Geometry: see drawing. Coordinates: mm, zero at the bounding-box minimum. A direction names the side the tool comes from. Coordinates: 2 decimals unless noted, no trailing zeros. Loops run counter-clockwise (first coordinate to the right, second up) from the corner with the lowest first, then second, coordinate; pieces in that order, holes last. Notation, with made-up numbers: (73, 11.25) -> (86, 11.25) arc R15 cw to (86, 16.25) -> close; hole circle Ø3 at (-25.5, 64.5). An arc over 180 degrees is marked (long way). Answer as a JSON object with one key per item and string values.
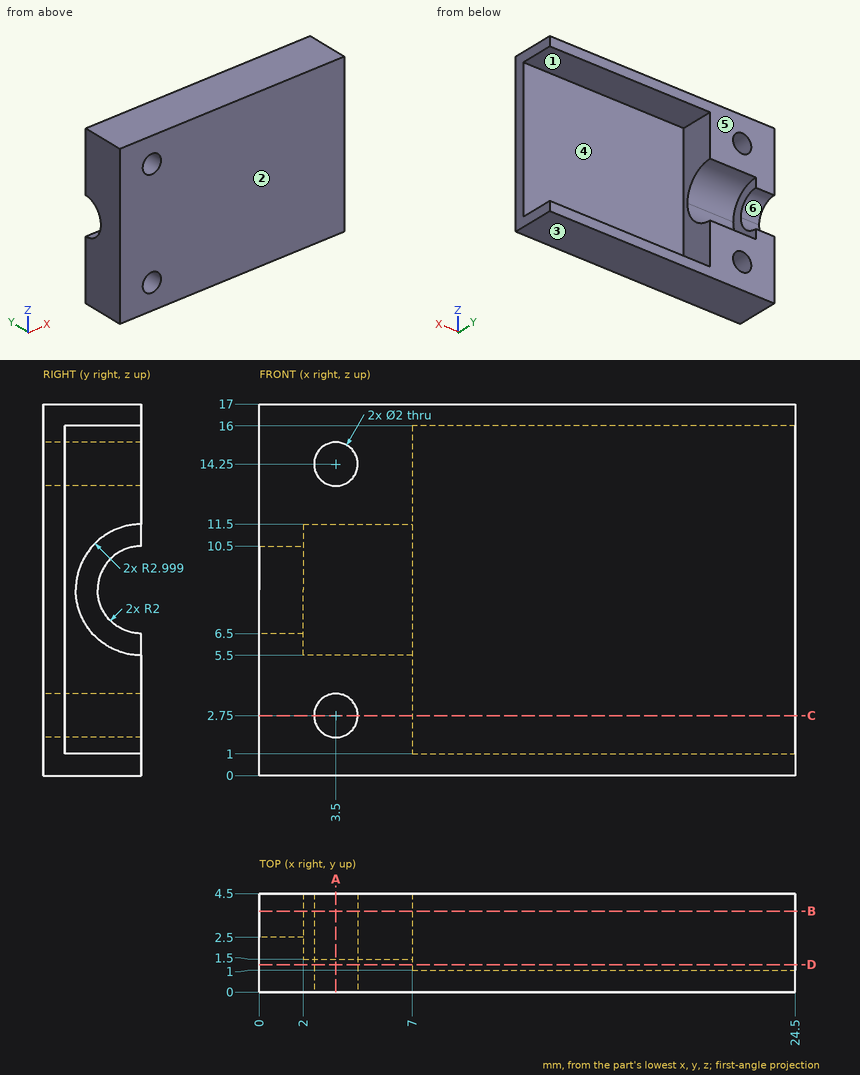
1. Line query: line 1 along Z through (x, y) = (3.5, 0.9); line 2 along X through (y, z) = (2.3, 14.25); line 3 along Z through (x, y) = (3.5, 2.1). Output: solid intervals per line, ascending.
Reply:
{"line 1": "z = 0 to 1.75, 3.75 to 13.25, 15.25 to 17", "line 2": "x = 0 to 2.5, 4.5 to 7", "line 3": "z = 0 to 1.75, 3.75 to 6.7, 10.3 to 13.25, 15.25 to 17"}
2. Section query D-D (y = 1.25). Return loops of the section in (x, z).
Reply:
{"outline": "(0, 0) -> (24.5, 0) -> (24.5, 1) -> (7, 1) -> (7, 16) -> (24.5, 16) -> (24.5, 17) -> (0, 17) -> close; hole circle Ø2 at (3.5, 2.75); hole circle Ø2 at (3.5, 14.25)"}
3. Section query B-B (y = 3.7). Return loops of the section in (x, z).
Reply:
{"outline": "(0, 0) -> (24.5, 0) -> (24.5, 1) -> (7, 1) -> (7, 5.61) -> (2, 5.61) -> (2, 6.67) -> (0, 6.67) -> close; (0, 10.33) -> (2, 10.33) -> (2, 11.39) -> (7, 11.39) -> (7, 16) -> (24.5, 16) -> (24.5, 17) -> (0, 17) -> close; hole circle Ø2 at (3.5, 2.75); hole circle Ø2 at (3.5, 14.25)"}
4. Pin query (flat end, axial travel): P1, Ø1.8, axis at y = 2, z = 8, coming from the +X side; P2, Ø3, axis at x = 3.5, z = 14.25, coming from the -Y side; P3, Ø4.5, axis at x = 12.5, z = 6, coming from the +Y side. Return the tip coordinate at first contact, or that it passes through.
Reply:
{"P1": "stops at x = 7", "P2": "stops at y = 0", "P3": "stops at y = 1"}
5. Access query for the marked faces 4, 5 and 6. Directions: +Z, -Z, +X, -X, +Y, -Y. A direction counts if a zero-diameter tool reaches every point of the face in a straight line with its end or side. Return the directions, or none.
Reply:
{"face 4": "+X, +Y", "face 5": "+Z, -Z, +X, -X, +Y", "face 6": "+X, -X, +Y"}
6. Mould query, pull axis Z, two halves, no side actions, for the marked faces 1, 2 and 3. Classes: pulls with the +Z half, pulls with the -Z half, needs draft (parallel to the pull), parting line crosses it, or undercut.
Reply:
{"face 1": "undercut", "face 2": "needs draft", "face 3": "pulls with the -Z half"}
7. Section query A-A (x = 3.5). Count the separate pieces of the cut face and the enclosed holes in it.
Reply:
{"separate pieces": "3", "enclosed holes": "0"}
8. Section query C-C (z = 2.75). Return loops of the section in (x, y).
Reply:
{"outline": "(0, 0) -> (2.5, 0) -> (2.5, 4.5) -> (0, 4.5) -> close; (4.5, 0) -> (24.5, 0) -> (24.5, 1) -> (7, 1) -> (7, 4.5) -> (4.5, 4.5) -> close"}
